```python
from build123d import *

# Parameters (mm, degrees)
SKETCH1_R           = 28.25
BOSS_EXTRUDE1_DEPTH = 41
SKETCH2_R           = 26.75
CUT_EXTRUDE1_DEPTH  = 39.5
SKETCH3_R           = 9.075
SKETCH3_R_2         = 7.575
BOSS_EXTRUDE2_DEPTH = 3.5
SKETCH4_R           = 9.075
SKETCH4_R_2         = 6.775
BOSS_EXTRUDE3_DEPTH = 1.5
SKETCH5_R           = 7.575
CUT_EXTRUDE2_DEPTH  = 1.5
SKETCH6_W           = 4
SKETCH6_H           = 4
BOSS_EXTRUDE4_DEPTH = 3.5
CUT_EXTRUDE3_DEPTH  = 37.5
FILLET1_R           = 1
FILLET1_2_R         = 0.5


with BuildPart() as part:
    # Sketch1 → Boss-Extrude1 (new body)
    with BuildSketch(Plane(origin=(0, 0, 0), x_dir=(1, 0, 0), z_dir=(0, 1, 0))):
        Circle(SKETCH1_R)
    extrude(amount=BOSS_EXTRUDE1_DEPTH)

    # Sketch2 → Cut-Extrude1 (cut)
    with BuildSketch(Plane.XZ):
        Circle(SKETCH2_R)
    extrude(amount=-CUT_EXTRUDE1_DEPTH, mode=Mode.SUBTRACT)

    # Sketch3 → Boss-Extrude2 (add)
    with BuildSketch(Plane(origin=(0, 41, 0), x_dir=(1, 0, 0), z_dir=(0, 1, 0))):
        Circle(SKETCH3_R)
        Circle(SKETCH3_R_2, mode=Mode.SUBTRACT)
    extrude(amount=BOSS_EXTRUDE2_DEPTH)

    # Sketch4 → Boss-Extrude3 (add)
    with BuildSketch(Plane(origin=(0, 44.5, 0), x_dir=(1, 0, 0), z_dir=(0, 1, 0))):
        Circle(SKETCH4_R)
        Circle(SKETCH4_R_2, mode=Mode.SUBTRACT)
    extrude(amount=-BOSS_EXTRUDE3_DEPTH)

    # Sketch5 → Cut-Extrude2 (cut)
    with BuildSketch(Plane(origin=(0, 41, 0), x_dir=(1, 0, 0), z_dir=(0, 1, 0))):
        Circle(SKETCH5_R)
    extrude(amount=-CUT_EXTRUDE2_DEPTH, mode=Mode.SUBTRACT)

    # Sketch6 → Boss-Extrude4 (add)
    with BuildSketch(Plane(origin=(0, 44.5, 0), x_dir=(1, 0, 0), z_dir=(0, 1, 0))):
        with Locations((0, -10.851871271)):
            Rectangle(SKETCH6_W, SKETCH6_H)
    extrude(amount=-BOSS_EXTRUDE4_DEPTH)

    # Sketch8 → Cut-Extrude3 (cut)
    with BuildSketch(Plane.XZ):
        with BuildLine():
            Line((-18.827156573, -21.06182982), (-16.65, -12.936570875))
            Line((-16.65, -12.936570875), (-16.65, 12.95))
            Line((-16.65, 12.95), (16.65, 12.95))
            Line((16.65, 12.95), (16.65, -12.936570875))
            Line((16.65, -12.936570875), (18.827156573, -21.06182982))
            ThreePointArc((18.827156573, -21.06182982), (0, -28.25), (-18.827156573, -21.06182982))
        make_face()
    extrude(amount=-CUT_EXTRUDE3_DEPTH, mode=Mode.SUBTRACT)

    # Fillet1
    fillet1_edges = [part.edges().sort_by_distance(p)[0] for p in [
        (-2, 42.75, 12.851871271),
        (2, 42.75, 12.851871271),
        (-28.25, 41, 0),
    ]]
    fillet(fillet1_edges, radius=FILLET1_R)

    # Fillet1 2
    fillet1_2_edges = [part.edges().sort_by_distance(p)[0] for p in [
        (0, 44.5, -9.075),
        (-2, 44.5, 10.851871271),
        (0, 44.5, 12.851871271),
        (2, 44.5, 10.851871271),
    ]]
    fillet(fillet1_2_edges, radius=FILLET1_2_R)


solid = part.part
```
The model under review builds one solid part; all positions refer to its coordinate system, in mm. A direction names the side the tool comes from. Round coordinates to 2 decimals unless told otherwise and drop trailing zeros. Write each loop counter-clockwise with the first axis right and the second up, starting at its lowest first coordinate (ties: lowest second). Pieces come first, ordered by that corner, then holes.
(1) Insertion check: pin 1 (15.5 mm diameter, centred on x = 0, z = 0, fed in from -Y); pin 2 (6 mm diameter, centred on x = 13, z = 15.5, fed in from +Y); pin 3 (1 mm diameter, centred on x = -6.5, y = 9, fed in from -Z). Each pin has a flat end and moves straight along its axis. Give the tip position at first contact, or say it passes through.
(2) Wall thickness on L1, parallel to X at y = 12, z = 0; L2, parallel to Y at x = -23, z = -13; L3, parallel to X at y = 42, z = 0 (3 decimals): over which ranges is each line inside the solid? List them lowest first.
(3) We need section A-A on x = 0. Give the boundary of the cut face in (y, z) (3 decimals).
(4) Mouldability with a two-part tool opening along Z and no side actions: class faces 4 (the flat face through (-18.611, 18.488, -20.256)), 5 (the flat face through (6, 39.5, -6)), 6 (the cylindrical face through (-6.01, 41.23, 4.61)), 7 (the flat face through (12, 41, 0)) as +Z half, -Z half, draft (parallel to the pull), parting line (faces both ways), or undercut.
(5) Machinability: for faces 1 (the flat face through (18.605, 18.488, -20.233)), 2 (the flat face through (-6, 43, 4)), 3 (the cylindrical face through (0.371, 42.479, -9.067)), which of the approach directions +Z, -Z, +X, -X, +Y, -Y give a long, thin tool a straight path to every point of the face, cutting with its end or side? Answer none if there is none.
(6) We need section C-C on y = 16.5. Give the boundary of the cut face in (x, z).
(7) We need section B-B on z = 0. Give the boundary of the cut face in (x, y) (3 decimals).
Findings below:
1. pin 1: stops at y = 39.5
1. pin 2: stops at y = 41
1. pin 3: stops at z = 25.82
2. L1: x = -28.25 to -26.75, 26.75 to 28.25
2. L2: y = 39.5 to 41
2. L3: x = -9.075 to -7.575, 7.575 to 9.075
3. outline: (0, 26.75) - (39.5, 26.75) - (39.5, 7.575) - (43, 7.575) - (43, 6.775) - (44.5, 6.775) - (44.5, 12.352) arc R0.5 ccw to (44, 12.852) - (41, 12.852) - (41, 27.25) arc R1 ccw to (40, 28.25) - (0, 28.25) - close; (37.5, -28.25) - (40, -28.25) arc R1 ccw to (41, -27.25) - (41, -9.075) - (44, -9.075) arc R0.5 ccw to (44.5, -8.575) - (44.5, -6.775) - (43, -6.775) - (43, -7.575) - (39.5, -7.575) - (39.5, -26.75) - (37.5, -26.75) - close
4. face 4: -Z half
4. face 5: undercut
4. face 6: undercut
4. face 7: draft
5. face 1: -Z, -Y
5. face 2: -Y
5. face 3: +Y
6. outline: (-18.83, -21.06) - (-18.39, -19.43) arc R26.75 cw (long way) to (18.39, -19.43) - (18.83, -21.06) arc R28.25 ccw (long way) to start
7. outline: (-28.25, 0) - (-26.75, 0) - (-26.75, 39.5) - (-7.575, 39.5) - (-7.575, 43) - (-6.775, 43) - (-6.775, 44.5) - (-8.575, 44.5) arc R0.5 ccw to (-9.075, 44) - (-9.075, 41) - (-27.25, 41) arc R1 ccw to (-28.25, 40) - close; (6.775, 43) - (7.575, 43) - (7.575, 39.5) - (26.75, 39.5) - (26.75, 0) - (28.25, 0) - (28.25, 40) arc R1 ccw to (27.25, 41) - (9.075, 41) - (9.075, 44) arc R0.5 ccw to (8.575, 44.5) - (6.775, 44.5) - close
